For this review, take the finished solid that the model builds, in its own axes (mm). Face numbers are marked on the shaded views. A direction names the side the tool comes from. Give positions to 0.01 mm unless a question says otherwise; leave off trailing zeros. Order: outer loops, then holes, each group sorted by start corner. A loop starts at its lowest first (then second) coordinate and runs counter-clockwise, first axis right, second up. Notation, with made-up numbers: (82.25, 0.5) -> (108.25, 0.5) arc R4 cw to (108.25, 6.5) -> close; hole circle Ø6 at (-16.75, 66). An arc over 180 degrees is marked (long way). Use CSV: the item, a comma, the result in double quotes. Start each with the question number.
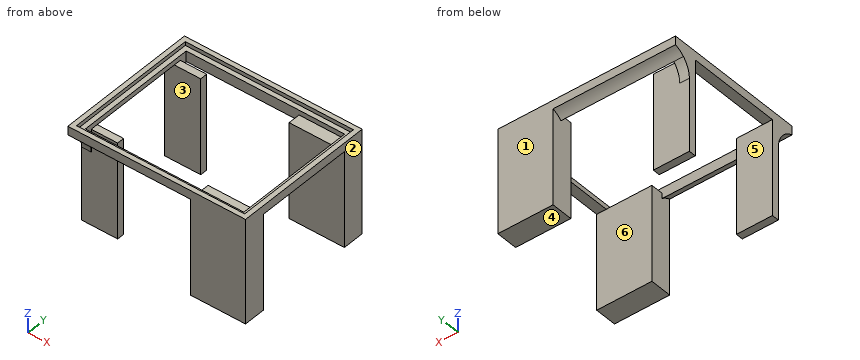
```python
from build123d import *

# Parameters (mm, degrees)
SKETCH1_W                = 70
SKETCH1_H                = 55
SKETCH1_W_2              = 66
SKETCH1_H_2              = 51
BOSS_EXTRUDE1_DEPTH      = 2
BOSS_EXTRUDE2_DEPTH      = 1.6
BOSS_EXTRUDE2_DEPTH_BACK = 2
SKETCH2_W                = 74
SKETCH2_H                = 59
SKETCH2_W_2              = 70
SKETCH2_H_2              = 55
SKETCH3_W                = 23
SKETCH3_H                = 9
SKETCH3_W_2              = 15
SKETCH3_H_2              = 3
BOSS_EXTRUDE3_DEPTH      = 40
FILLET1_START            = -37
FILLET1_DEPTH            = 70
FILLET1_2_DEPTH          = 4


with BuildPart() as part:
    # Sketch1 → Boss-Extrude1 (new body)
    with BuildSketch(Plane.XY):
        Rectangle(SKETCH1_W, SKETCH1_H)
        Rectangle(SKETCH1_W_2, SKETCH1_H_2, mode=Mode.SUBTRACT)
    extrude(amount=BOSS_EXTRUDE1_DEPTH)

    # Sketch2 → Boss-Extrude2 (add, two sides: drawn at the far end of the back side and taken through both)
    with BuildSketch(Plane.XY.offset(2).offset(-BOSS_EXTRUDE2_DEPTH_BACK)):
        Rectangle(SKETCH2_W, SKETCH2_H)
        Rectangle(SKETCH2_W_2, SKETCH2_H_2, mode=Mode.SUBTRACT)
    extrude(amount=BOSS_EXTRUDE2_DEPTH + BOSS_EXTRUDE2_DEPTH_BACK)

    # Sketch3 → Boss-Extrude3 (add)
    with BuildSketch(Plane(origin=(0, 0, 0), x_dir=(-1, 0, 0), z_dir=(0, 0, -1))):
        with Locations((-25.5, 25)):
            Rectangle(SKETCH3_W, SKETCH3_H)
        with Locations((-25.5, -25)):
            Rectangle(SKETCH3_W, SKETCH3_H)
        with Locations((29.5, 21)):
            Rectangle(SKETCH3_W_2, SKETCH3_H_2)
        with Locations((29.5, -21)):
            Rectangle(SKETCH3_W_2, SKETCH3_H_2)
    extrude(amount=BOSS_EXTRUDE3_DEPTH)

    # Fillet1: read off the stored shape, not the designer's step
    # Fillet1 outline → Fillet1 (add)
    with BuildSketch(Plane.YZ.offset(FILLET1_START)):
        with BuildLine():
            Line((29.5, 0), (25.5, 0))
            Line((25.5, 0), (25.5, -2.397963586))
            ThreePointArc((25.5, -2.397963586), (27.358253474, -0.962536958), (29.5, 0))
        make_face()
        with BuildLine():
            ThreePointArc((-29.5, 0), (-27.358253474, -0.962536958), (-25.5, -2.397963586))
            Line((-25.5, -2.397963586), (-25.5, 0))
            Line((-25.5, 0), (-29.5, 0))
        make_face()
    extrude(amount=FILLET1_DEPTH)

    # Fillet1 2 outline → Fillet1 2 (add)
    with BuildSketch(Plane.YZ.offset(FILLET1_START)):
        with BuildLine():
            Line((25.5, -2.397963586), (25.5, 0))
            Line((25.5, 0), (22.5, 0))
            Line((22.5, 0), (22.5, -9.539392014))
            ThreePointArc((22.5, -9.539392014), (23.280455543, -5.666408668), (25.5, -2.397963586))
        make_face()
        with BuildLine():
            Line((-25.5, 0), (-25.5, -2.397963586))
            ThreePointArc((-25.5, -2.397963586), (-23.280455543, -5.666408668), (-22.5, -9.539392014))
            Line((-22.5, -9.539392014), (-22.5, 0))
            Line((-22.5, 0), (-25.5, 0))
        make_face()
    extrude(amount=FILLET1_2_DEPTH)


solid = part.part
```
1. Draft analysis for pull direction Y (two halves, no side actions). For the marked faces 1, 2 and 3, state which applies: +Y half, -Y half, draft (parallel to the pull), parting line (faces both ways), or undercut.
2. Clearance check with flat-ended pins moving along their axes: P1, Ø2.5, axis at x = 22, y = -23, coming from the +Z side; P2, Ø7, axis at y = -26.5, z = -15, coming from the -X side; P3, Ø4, axis at x = -23.5, z = -24.5, coming from the +Y side. State where each tip first meets the part, or that it passes through.
3. Consider section A-A (z = -19). State the section outline as (x, y) points, plus the area to 3 significant figures.
4. Consider section B-B (x = -15). State the section outline as (y, z) points.
5. To check wall thickness, follow L1, parallel to Y at x = 25, z = -10.5; L2, parallel to X at y = 21, z = -3.5; L3, parallel to Y at x = -24, z = -21. State the ranges of each line that lie inside material, in increasing order. Write a range as [from, to].
6. For the marked faces 4, 5 and 6, list the 3-axis set-ups (+Z, -Z, +X, -X, +Y, -Y) from which the entire face can be reached by the end or side of a thin tool; tool diameter is ignored.
7. Consider section C-C (y = -12). State the section outline as (x, z) points, plus the area to 3 significant figures.
8. Consider section D-D (x = -30.5). State the section outline as (y, z) points, plus the area to 3 significant figures.
Answer list:
1,face 1,"+Y half"
1,face 2,"draft"
1,face 3,"undercut"
2,P1,"z = 0"
2,P2,"x = 14"
2,P3,"y = 22.5"
3,outline,"(-37, -22.5) -> (-22, -22.5) -> (-22, -19.5) -> (-37, -19.5) -> close; (-37, 19.5) -> (-22, 19.5) -> (-22, 22.5) -> (-37, 22.5) -> close; (14, -29.5) -> (37, -29.5) -> (37, -20.5) -> (14, -20.5) -> close; (14, 20.5) -> (37, 20.5) -> (37, 29.5) -> (14, 29.5) -> close"
3,area,"504 mm2"
4,outline,"(-29.5, 0) arc R10 cw to (-25.5, -2.4) -> (-25.5, 2) -> (-27.5, 2) -> (-27.5, 3.6) -> (-29.5, 3.6) -> close; (25.5, -2.4) arc R10 cw to (29.5, 0) -> (29.5, 3.6) -> (27.5, 3.6) -> (27.5, 2) -> (25.5, 2) -> close"
5,L1,"[-29.5, -20.5], [20.5, 29.5]"
5,L2,"[-37, -22], [14, 37]"
5,L3,"[-22.5, -19.5], [19.5, 22.5]"
6,face 4,"-Z, +X, -X, +Y, -Y"
6,face 5,"-Z, +X, -X"
6,face 6,"-Z, +X"
7,outline,"(-37, 0) -> (-33, 0) -> (-33, 2) -> (-35, 2) -> (-35, 3.6) -> (-37, 3.6) -> close; (33, 0) -> (37, 0) -> (37, 3.6) -> (35, 3.6) -> (35, 2) -> (33, 2) -> close"
7,area,"22.4 mm2"
8,outline,"(-29.5, 0) arc R10 cw to (-25.5, -2.4) -> (-25.5, 2) -> (-27.5, 2) -> (-27.5, 3.6) -> (-29.5, 3.6) -> close; (-22.5, -40) -> (-19.5, -40) -> (-19.5, 0) -> (-22.5, 0) -> close; (19.5, -40) -> (22.5, -40) -> (22.5, 0) -> (19.5, 0) -> close; (25.5, -2.4) arc R10 cw to (29.5, 0) -> (29.5, 3.6) -> (27.5, 3.6) -> (27.5, 2) -> (25.5, 2) -> close"
8,area,"270 mm2"
